Read the model definition and answer for the solid it produces. Units are mm, in the model's axes. Give positions to 0.01 mm unless a question says otherwise; leave off trailing zeros. Write each loop counter-clockwise with the first axis right and the second up, starting at its lowest first coordinate (ties: lowest second). Pieces come first, ordered by that corner, then holes. Notation, with made-up numbers: (-13.5, 41) -> (16.5, 41) arc R10 cw to (16.5, 52) -> close; hole circle Ø10 at (31, 53.25). An arc over 180 degrees is marked (long way). Use a Markdown table: item, result.
from build123d import *

# Parameters (mm, degrees)
F5_DEPTH = 4
F7_D     = 3
F9_DEPTH = 4.001


with BuildPart() as f5:
    # F4 (on Top) → F5 (new body)
    with BuildSketch(Plane.XY):
        Polygon((31.7157287525, 60), (-31.7157287525, 60), (-45.8578643763, 45.8578643763), (-60, 31.7157287525), (-53.459262274, 24.1143308548), (-52.5, 22.9995125363), (-52.5, -22.9995125363), (-60, -31.7157287525), (-45.8578643763, -45.8578643763), (-31.7157287525, -60), (31.7157287525, -60), (45.8578643763, -45.8578643763), (60, -31.7157287525), (52.5, -22.9995125363), (52.5, 22.9995125363), (60, 31.7157287525), (45.8578643763, 45.8578643763), align=None)
    extrude(amount=F5_DEPTH)

    # F7 (through all)
    with Locations(Plane(origin=(0, 0, 0), x_dir=(1, 0, 0), z_dir=(0, 0, -1))):
        with Locations((-49.3933982822, -35.2512626585), (-35.2512626585, -49.3933982822), (35.5175525155, -49.6500174851), (49.1271084251, -34.9946434556), (49.3933982822, 35.2512626585), (35.2512626585, 49.3933982822), (-35.2512626585, 49.3933982822), (-49.3933982822, 35.2512626585)):
            Hole(F7_D / 2)

    # F8 (on face) + F0 (on Top) → F9 (cut, through all)
    with BuildSketch(Plane.XY.offset(4)):
        with BuildLine():
            ThreePointArc((-20.5, 42.5), (-22.5, 44.5), (-24.5, 42.5))
            Line((-24.5, 42.5), (-24.5, 17.5))
            ThreePointArc((-24.5, 17.5), (-22.5, 15.5), (-20.5, 17.5))
            Line((-20.5, 17.5), (-20.5, 42.5))
        make_face()
        with BuildLine():
            ThreePointArc((24.5, 42.5), (22.5, 44.5), (20.5, 42.5))
            Line((20.5, 42.5), (20.5, 17.5))
            ThreePointArc((20.5, 17.5), (22.5, 15.5), (24.5, 17.5))
            Line((24.5, 17.5), (24.5, 42.5))
        make_face()
        with BuildLine():
            ThreePointArc((20.5, -42.5), (22.5, -44.5), (24.5, -42.5))
            Line((24.5, -42.5), (24.5, -17.5))
            ThreePointArc((24.5, -17.5), (22.5, -15.5), (20.5, -17.5))
            Line((20.5, -17.5), (20.5, -42.5))
        make_face()
        with BuildLine():
            ThreePointArc((-20.5, -17.5), (-22.5, -15.5), (-24.5, -17.5))
            Line((-24.5, -17.5), (-24.5, -42.5))
            ThreePointArc((-24.5, -42.5), (-22.5, -44.5), (-20.5, -42.5))
            Line((-20.5, -42.5), (-20.5, -17.5))
        make_face()
    with BuildSketch(Plane.XY):
        with BuildLine():
            Line((-92.5269119346, 112.3259018078), (-120.6951909025, 148.176438676))
            ThreePointArc((-120.6951909025, 148.176438676), (-118.5238761033, 143.1793796454), (-117.7817459305, 137.7817459305))
            ThreePointArc((-117.7817459305, 137.7817459305), (-127.9810789866, 120.3476721824), (-148.176438676, 120.6951909025))
            Line((-148.176438676, 120.6951909025), (-112.3259018078, 92.5269119346))
            Line((-112.3259018078, 92.5269119346), (-60, 31.7157287525))
            Line((-60, 31.7157287525), (-31.7157287525, 60))
            Line((-31.7157287525, 60), (-92.5269119346, 112.3259018078))
        make_face()
    extrude(amount=-F9_DEPTH, mode=Mode.SUBTRACT)


solid = f5.part
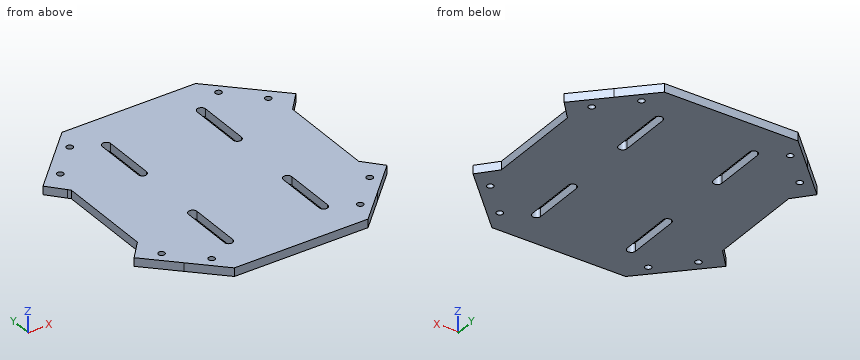
Item 1: Each of these flat-tipped pins is pushed along its axis until it touches: P1, Ø2.5, axis at x = -49.39, y = -35.25, coming from the -Z side; P2, Ø2, axis at y = 28.5, z = 2.5, coming from the +X side; P3, Ø2, axis at y = 2, z = 2.5, coming from the -X side; P4, Ø2, axis at y = 26.5, z = 1.5, coming from the +X side. Where does it stop, or does it pass through?
Return value:
| item | result |
|---|---|
| P1 | through |
| P2 | x = 58.09 |
| P3 | x = -52.5 |
| P4 | x = 56.37 |
Item 2: A cutting plane is placed at C-C (z = 3.2). Count the separate pieces of the cut face and the enclosed holes in it, then the cut area to 3 significant figures.
Return value:
| item | result |
|---|---|
| separate pieces | 1 |
| enclosed holes | 12 |
| area | 11,500 mm^2 |
Item 3: A cutting plane is placed at B-B (y = -5). Give the vertices of the cut face in (x, z), then the cut area to 3 significant figures.
Return value:
| item | result |
|---|---|
| outline | (-52.5, 0) -> (52.5, 0) -> (52.5, 4) -> (-52.5, 4) -> close |
| area | 420 mm^2 |
Item 4: Straight lines are drawn through the part: line 1 along X through (y, z) = (50.5, 3); line 2 along X through (y, z) = (-29, 1.15); line 3 along X through (y, z) = (13, 2.1). For each, find the intervals that lie inside material, in ascending order. Write a range as [from, to].
Return value:
| item | result |
|---|---|
| line 1 | [-41.22, -36.26], [-34.24, 34.28], [36.75, 41.22] |
| line 2 | [-57.66, -24.5], [-20.5, 20.5], [24.5, 57.66] |
| line 3 | [-52.5, 52.5] |
Item 5: A cutting plane is placed at A-A (x = 22.5). Give the vertices of the cut face in (y, z), then the cut area to 3 significant figures.
Return value:
| item | result |
|---|---|
| outline | (-60, 0) -> (-44.5, 0) -> (-44.5, 4) -> (-60, 4) -> close; (-15.5, 0) -> (15.5, 0) -> (15.5, 4) -> (-15.5, 4) -> close; (44.5, 0) -> (60, 0) -> (60, 4) -> (44.5, 4) -> close |
| area | 248 mm^2 |
